Work out the finished part from the listing and answer in its coordinate system (mm). A direction names the side the tool comes from. Coordinates: 2 decimals unless noted, no trailing zeros. Order: outer loops, then holes, each group sorted by start corner. A loop starts at its lowest first (then second) coordinate and runs counter-clockwise, first axis right, second up. Notation, with made-up numbers: M 74.25,-35.75 L 132.25,-35.75 A17 ccw 132.25,-13.75 Z; hole C 79.5,-15 d2. An arc over 180 degrees is marked long. Use a Markdown table: item, result.
from build123d import *

# Parameters (mm, degrees)
F0_W     = 25.4
F0_H     = 25.4
F1_DEPTH = 12.7
F2_W     = 19.05
F2_H     = 19.05
F3_DEPTH = 6.35
F4_W     = 12.7
F4_H     = 12.7
F5_DEPTH = 6.35


with BuildPart() as f1:
    # F0 (on Top) → F1 (new body)
    with BuildSketch(Plane.XY):
        Rectangle(F0_W, F0_H)
    extrude(amount=F1_DEPTH)

    # F2 (on face) → F3 (join)
    with BuildSketch(Plane.XY.offset(12.7)):
        Rectangle(F2_W, F2_H)
    extrude(amount=F3_DEPTH)

    # F4 (on face) → F5 (join)
    with BuildSketch(Plane.XY.offset(19.05)):
        Rectangle(F4_W, F4_H)
    extrude(amount=F5_DEPTH)


solid = f1.part
(1) Which of the six approach directions +Z, -Z, +X, -X, +Y, -Y give full straight-line access (tool end or side, diameter ignored) to faces 4 (the flat face through (-6.35, 0, 22)), 5 (the flat face through (0, 6.35, 22)), 6 (the flat face through (0, -6.35, 22)), 7 (the flat face through (9.525, 0, 16))?
Conclusion:
| item | result |
|---|---|
| face 4 | +Z, -X, +Y, -Y |
| face 5 | +Z, +X, -X, +Y |
| face 6 | +Z, +X, -X, -Y |
| face 7 | +Z, +X, +Y, -Y |
(2) A cutting plane is placed at A-A (y = -8.75). Determine the outline of the cut face in (x, z) (3 decimals), then the cut area to 3 significant figures.
Conclusion:
| item | result |
|---|---|
| outline | M -12.7,0 L 12.7,0 L 12.7,12.7 L 9.525,12.7 L 9.525,19.05 L -9.525,19.05 L -9.525,12.7 L -12.7,12.7 Z |
| area | 444 mm2 |
(3) A cutting plane is placed at C-C (y = 3.5). Determine the outline of the cut face in (x, z) (3 decimals), then the cut area to 3 significant figures.
Conclusion:
| item | result |
|---|---|
| outline | M -12.7,0 L 12.7,0 L 12.7,12.7 L 9.525,12.7 L 9.525,19.05 L 6.35,19.05 L 6.35,25.4 L -6.35,25.4 L -6.35,19.05 L -9.525,19.05 L -9.525,12.7 L -12.7,12.7 Z |
| area | 524 mm2 |
(4) Given P1, Ø1.9, axis at y = 1.5, z = 14.5, coming from the -X side (3 decimals); P2, Ø3, axis at y = 1.5, z = 22, coming from the -X side; P3, Ø3, axis at x = -0.5, z = 15, coming from the +Y side (3 decimals), each flat-ended and moving along its own axis, determine where each tip first touches the part or whether it passes through.
Conclusion:
| item | result |
|---|---|
| P1 | x = -9.525 |
| P2 | x = -6.35 |
| P3 | y = 9.525 |
(5) Straight lines are drawn through the part: L1, parallel to X at y = 5.75, z = 21; L2, parallel to Z at x = 2, y = -9.75. For each, find the intervals that lie inside material, in ascending order.
Conclusion:
| item | result |
|---|---|
| L1 | -6.35 to 6.35 |
| L2 | 0 to 12.7 |
(6) Determine the mould class of faces 1 (the flat face through (0, -9.525, 16)), 2 (the flat face through (-12.7, 0, 6)), 3 (the flat face through (6.35, 0, 22)) for opening direction X: pulls with the +X half, pulls with the -X half, needs draft (parallel to the pull), parting line crosses it, or undercut.
Conclusion:
| item | result |
|---|---|
| face 1 | needs draft |
| face 2 | pulls with the -X half |
| face 3 | pulls with the +X half |
(7) A cutting plane is placed at D-D (z = 23.75). Determine the outline of the cut face in (x, y), then the cut area to 3 significant figures.
Conclusion:
| item | result |
|---|---|
| outline | M -6.35,-6.35 L 6.35,-6.35 L 6.35,6.35 L -6.35,6.35 Z |
| area | 161 mm2 |
